Source: CAD feature listing. Evaluate the final solid. Frame: model axes, mm. Give positions to 0.01 mm unless a question says otherwise; leave off trailing zeros. Order: outer loops, then holes, each group sorted by start corner. A loop starts at its lowest first (then second) coordinate and runs counter-clockwise, first axis right, second up. Notation, with made-up numbers: (63.5, -11.5) - (115.5, -11.5) arc R27 cw to (115.5, 27.5) - close; hole circle Ø7 at (41, 40.25). An arc over 180 degrees is marked (long way). Write each question's results on one line, items separated by ' | '. Start each with the question number.
Item 1: Section A-A on y = -2.42. Output: boundary loops of the cut face in (x, z), and give its area (3 significant figures).
Item 2: Section C-C on z = 4.25. Output: boundary loops of the cut face in (x, y), and give its area (3 significant figures).
Item 3: Section B-B on x = 3.5. Output: boundary loops of the cut face in (y, z).
Item 4: Line query: line 1 along X through (y, z) = (-0.8, -0.25); line 2 along Y through (x, z) = (1.5, 7.5); line 3 along Z through (x, y) = (4.25, -2.3). Output: solid intervals per line, ascending.
Item 5: Contact query for flat-ended pins moving along their axis: pin 1 Ø0.9 at (y, z) = (-3, 0) entering from -X; pin 2 Ø0.6 at (x, y) = (0, -2) entering from -Z; pin 3 Ø1.3 at (x, y) = (6, -2) entering from -Z. Output: stop coordinate, or through.
Item 6: Mould query, pull axis X, two halves, no side actions, for faces 1 (the flat face through (9.02, -2.4, -0.2)), 2 (the flat face through (0, -2, 4)), 3 (the flat face through (5, 0, 5)). Classes: released by +X, released by -X, zero draft, split by the parting line, or undercut.
Item 7: Section D-D on y = -0.35. Output: boundary loops of the cut face in (x, z), and give its area (3 significant figures).
```python
from build123d import *

# Parameters (mm, degrees)
SKETCH_W     = 9.53
SKETCH_H     = 9.52
PAD_DEPTH    = 4.44
SKETCH001_W  = 0.51
SKETCH001_H  = 0.81
PAD001_DEPTH = 4.83
SKETCH004_R  = 0.255
PAD003_DEPTH = 6.86


with BuildPart() as part:
    # Sketch → Pad (new body)
    with BuildSketch(Plane.XZ):
        with Locations((4.765, 4.76)):
            Rectangle(SKETCH_W, SKETCH_H)
    extrude(amount=PAD_DEPTH)

    # Sketch001 → Pad001 (join)
    with BuildSketch(Plane.XZ):
        with Locations((0.255, 9.115)):
            Rectangle(SKETCH001_W, SKETCH001_H)
        with Locations((9.275, 9.115)):
            Rectangle(SKETCH001_W, SKETCH001_H)
        with Locations((9.275, -0.055)):
            Rectangle(SKETCH001_W, SKETCH001_H)
        with Locations((0.255, -0.055)):
            Rectangle(SKETCH001_W, SKETCH001_H)
    extrude(amount=PAD001_DEPTH)

    # Sketch004 (on Face19 of Pad001) → Pad003 (join)
    with BuildSketch(Plane(origin=(0, 0, 0), x_dir=(1, 0, 0), z_dir=(0, 0, -1))):
        with Locations((2.225, 2.42)):
            Circle(SKETCH004_R)
        with Locations((4.765, 2.42)):
            Circle(SKETCH004_R)
        with Locations((7.305, 2.42)):
            Circle(SKETCH004_R)
    extrude(amount=PAD003_DEPTH)


solid = part.part
```
Evaluation:
1) outline: (0, -0.46) - (0.51, -0.46) - (0.51, 0) - (1.97, 0) - (1.97, -6.86) - (2.48, -6.86) - (2.48, 0) - (4.51, 0) - (4.51, -6.86) - (5.02, -6.86) - (5.02, 0) - (7.05, 0) - (7.05, -6.86) - (7.56, -6.86) - (7.56, 0) - (9.02, 0) - (9.02, -0.46) - (9.53, -0.46) - (9.53, 9.52) - (0, 9.52) - close | area: 102 mm^2
2) outline: (0, -4.44) - (9.53, -4.44) - (9.53, 0) - (0, 0) - close | area: 42.3 mm^2
3) outline: (-4.44, 0) - (0, 0) - (0, 9.52) - (-4.44, 9.52) - close
4) line 1: x = 0 to 0.51, 9.02 to 9.53 | line 2: y = -4.44 to 0 | line 3: z = 0 to 9.52
5) pin 1: stops at x = 0 | pin 2: stops at z = -0.46 | pin 3: stops at z = 0
6) face 1: undercut | face 2: released by -X | face 3: zero draft
7) outline: (0, -0.46) - (0.51, -0.46) - (0.51, 0) - (9.02, 0) - (9.02, -0.46) - (9.53, -0.46) - (9.53, 9.52) - (0, 9.52) - close | area: 91.2 mm^2
